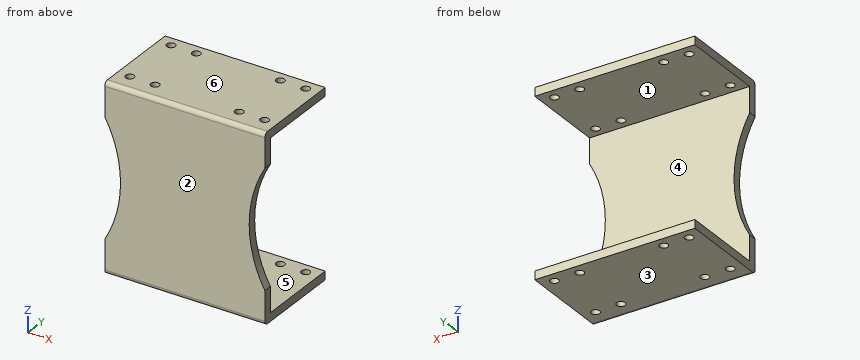
```python
from build123d import *

# Parameters (mm, degrees)
EXTRUDE_1_DEPTH     = 38
CUT_EXTRUDE_1_DEPTH = 38
SKETCH_4_R          = 1
CUT_EXTRUDE_3_DEPTH = 68
FILLET_1_R          = 1


with BuildPart() as part:
    # ｽｹｯﾁ1 → ﾎﾞｽ - 押し出し1 (new body)
    with BuildSketch(Plane(origin=(0, 0, 0), x_dir=(0, 0, -1), z_dir=(1, 0, 0))):
        Polygon((-22, 0), (22, 0), (22, 22), (20, 22), (20, 2), (-20, 2), (-20, 22), (-22, 22), align=None)
    extrude(amount=EXTRUDE_1_DEPTH)

    # ｽｹｯﾁ3 → ｶｯﾄ - 押し出し1 (cut)
    with BuildSketch(Plane(origin=(0, 12, 0), x_dir=(1, 0, 0), z_dir=(0, 1, 0))):
        with BuildLine():
            ThreePointArc((0, 14), (3.728865695, 0), (0, -14))
            Line((0, -14), (0, 14))
        make_face()
        with BuildLine():
            Line((38, 14), (38, -14))
            ThreePointArc((38, -14), (34.271134305, 0), (38, 14))
        make_face()
    extrude(amount=-CUT_EXTRUDE_1_DEPTH, mode=Mode.SUBTRACT)

    # ｽｹｯﾁ4 → ｶｯﾄ - 押し出し3 (cut)
    with BuildSketch(Plane.XY.offset(22)):
        with Locations((3.010351423, 19.5)):
            Circle(SKETCH_4_R)
        with Locations((9.033182751, 19.5)):
            Circle(SKETCH_4_R)
        with Locations(Location((3.010351423, 4.5, 0), (0, 0, 90))):
            Circle(SKETCH_4_R)
        with Locations(Location((9.033182751, 4.5, 0), (0, 0, 90))):
            Circle(SKETCH_4_R)
        with Locations(Location((28.966817249, 19.5, 0), (0, 0, 90))):
            Circle(SKETCH_4_R)
        with Locations(Location((34.989648577, 19.5, 0), (0, 0, 90))):
            Circle(SKETCH_4_R)
        with Locations((34.989648577, 4.5)):
            Circle(SKETCH_4_R)
        with Locations((28.966817249, 4.5)):
            Circle(SKETCH_4_R)
    extrude(amount=-CUT_EXTRUDE_3_DEPTH, mode=Mode.SUBTRACT)

    # ﾌｨﾚｯﾄ1
    fillet_1_edges = [part.edges().sort_by_distance(p)[0] for p in [
        (19, 0, 22),
        (19, 0, -22),
    ]]
    fillet(fillet_1_edges, radius=FILLET_1_R)


solid = part.part
```
Work out the finished part from the listing and answer in its coordinate system (mm). Face numbers are marked on the shaded views. A direction names the side the tool comes from. Give positions to 0.01 mm unless a question says otherwise; leave off trailing zeros. Loops run counter-clockwise (first coordinate to the right, second up) from the corner with the lowest first, then second, coordinate; pieces in that order, holes last. Notation, with made-up numbers: (4.25, 49) - (62.25, 49) arc R17 ccw to (62.25, 55) - close; hole circle Ø9 at (14.25, 11). An arc over 180 degrees is marked (long way). Use CSV: the item, a comma, the result in double quotes. Start each with the question number.
(1) Find the intervals of material crossed by L1, parallel to Z at x = 5.5, y = 14; L2, parallel to Y at x = 9.5, z = -19.5, in increasing order.
(2) Determine the mould class of the marked faces 3, 4, 5 and 6 for opening direction Z: released by +Z, released by -Z, zero draft, split by the parting line, or undercut.
(3) A tool of negligible diameter and unlimited length cuts with its end or side. For the marked faces 1 and 2, from which of +Z, -Z, +X, -X, +Y, -Y can it reach the whole face along a straight path? Write none if from no direction.
(4) Find section C-C, the plane z = 15.5. Determine the outline of the cut face in (x, y).
(5) Find section A-A, the plane y = 9.5. Determine the outline of the cut face in (x, z), plus the area to 3 significant figures.
(6) Find section B-B, the plane x = 5. Determine the outline of the cut face in (y, z), plus the area to 3 significant figures.
(7) Find section D-D, the plane y = 4.5. Count the separate pieces of the cut face and the enclosed holes in it, plus the area to 3 significant figures.
(8) Each of these flat-tipped pins is pushed along its axis until it touches: pin 1 (1.8 mm diameter, centred on x = 3.01, y = 19.5, fed in from -Z) (3 decimals); pin 2 (2.5 mm diameter, centred on x = 9.03, y = 4.5, fed in from -Z); pin 3 (1.5 mm diameter, centred on x = 9, z = 4.5, fed in from +Y). Where does it stop, or does it pass through?
Results found:
1,L1,"-22 to -20, 20 to 22"
1,L2,"0 to 2"
2,face 3,"released by -Z"
2,face 4,"undercut"
2,face 5,"undercut"
2,face 6,"released by +Z"
3,face 1,"+X, -X, +Y"
3,face 2,"+Z, -Z, +X, -X, -Y"
4,outline,"(0, 0) - (38, 0) - (38, 2) - (0, 2) - close"
5,outline,"(0, -22) - (38, -22) - (38, -20) - (0, -20) - close; (0, 20) - (38, 20) - (38, 22) - (0, 22) - close"
5,area,"152 mm^2"
6,outline,"(0, -21) arc R1 ccw to (1, -22) - (22, -22) - (22, -20) - (2, -20) - (2, 20) - (22, 20) - (22, 22) - (1, 22) arc R1 ccw to (0, 21) - close"
6,area,"168 mm^2"
7,separate pieces,"10"
7,enclosed holes,"0"
7,area,"120 mm^2"
8,pin 1,"through"
8,pin 2,"z = -22"
8,pin 3,"y = 2"
